from build123d import *

# Parameters (mm, degrees)
SKETCH_1_R          = 11
SKETCH_1_R_2        = 1.5
SKETCH_1_R_3        = 2
EXTRUDE_1_DEPTH     = 2
SKETCH_2_R          = 1
CUT_EXTRUDE_1_DEPTH = 10


with BuildPart() as part:
    # 草图1 → 凸台-拉伸1 (new body)
    with BuildSketch(Plane.XY):
        with Locations((-0.589945763, 5.342825614)):
            Circle(SKETCH_1_R)
        with Locations((-7.089945763, 1.842825614)):
            Circle(SKETCH_1_R_2, mode=Mode.SUBTRACT)
        with Locations(Location((5.910054237, 1.842825614, 0), (0, 0, 180))):
            Circle(SKETCH_1_R_2, mode=Mode.SUBTRACT)
        with Locations((-0.589945763, 1.842825614)):
            Circle(SKETCH_1_R_3, mode=Mode.SUBTRACT)
    extrude(amount=EXTRUDE_1_DEPTH)

    # 草图2 → 切除-拉伸1 (cut)
    with BuildSketch(Plane(origin=(0, 0, 0), x_dir=(-1, 0, 0), z_dir=(0, 0, -1))):
        with Locations((0.589945763, 16.342825614)):
            Circle(SKETCH_2_R)
    extrude(amount=-CUT_EXTRUDE_1_DEPTH, mode=Mode.SUBTRACT)


solid = part.part
Read the model definition and answer for the solid it produces. Units are mm, in the model's axes. Round coordinates to 2 decimals unless told otherwise and drop trailing zeros. Order: outer loops, then holes, each group sorted by start corner. A loop starts at its lowest first (then second) coordinate and runs counter-clockwise, first axis right, second up. Notation, with made-up numbers: (-32, 62) - (6, 62) arc R33 ccw to (6, 91) - close; hole circle Ø9 at (47, -37). An arc over 180 degrees is marked (long way). Use one line per item in the form item = value. Start each with the question number.
(1) The part is cut by section A-A (x = 5). Give the vertices of the cut face in (y, z), then the cut area to 3 significant figures.
(2) The part is cut by section D-D (x = -0.5). Give the vertices of the cut face in (y, z).
(3) A flat-ended cylindrical pin translates along its axis: pin 1 Ø12 at (x, y) = (3.5, 13.5) entering from -Z. Find the tip coordinate at first contact, or state that the pin passes through.
(4) The part is cut by section C-C (z = 0.8). Give the vertices of the cut face in (x, y).
(5) The part is cut by section B-B (y = 3). Give the vertices of the cut face in (x, z).
(6) Determine the mould class of faces 1 (the face through (-1.06, -5.647, 0.986)), 2 (the face through (-1, 5, 2)), 3 (the face through (7.41, 1.78, 0.99)) for opening direction X: +X half, -X half, draft (parallel to the pull), parting line (faces both ways), or undercut.
(7) Find the intervals of material crossed by line 1 along X through (y, z) = (5.25, 1.65); line 2 along Y through (x, z) = (-7, 0.9); line 3 along Y through (x, z) = (-2, 1.55), in increasing order. Write a range as from..to.
Checked values:
q1.outline = (-4.13, 0) - (0.65, 0) - (0.65, 2) - (-4.13, 2) - close; (3.04, 0) - (14.82, 0) - (14.82, 2) - (3.04, 2) - close
q1.area = 33.1 mm^2
q2.outline = (-5.66, 0) - (-0.16, 0) - (-0.16, 2) - (-5.66, 2) - close; (3.84, 0) - (15.35, 0) - (15.35, 2) - (3.84, 2) - close
q3.pin_1 = 0
q4.outline = (-1.59, 16.3) arc R11 ccw (long way) to (0.41, 16.3) arc R1 cw to start; hole circle Ø3 at (-7.09, 1.84); hole circle Ø4 at (-0.59, 1.84); hole circle Ø3 at (5.91, 1.84)
q5.outline = (-11.34, 0) - (-8.04, 0) - (-8.04, 2) - (-11.34, 2) - close; (-6.14, 0) - (-2.22, 0) - (-2.22, 2) - (-6.14, 2) - close; (1.04, 0) - (4.96, 0) - (4.96, 2) - (1.04, 2) - close; (6.86, 0) - (10.16, 0) - (10.16, 2) - (6.86, 2) - close
q6.face_1 = parting line
q6.face_2 = draft
q6.face_3 = undercut
q7.line_1 = -11.59..10.41
q7.line_2 = -3.6..0.35, 3.34..14.28
q7.line_3 = -5.57..0.42, 3.26..16.25
